Read the model definition and answer for the solid it produces. Units are mm, in the model's axes. Face numbers are marked on the shaded views. A direction names the side the tool comes from. Coordinates: 2 decimals unless noted, no trailing zeros. Loops run counter-clockwise (first coordinate to the right, second up) from the corner with the lowest first, then second, coordinate; pieces in that order, holes last. Notation, with made-up numbers: (-39.75, 20) - (-5.75, 20) arc R17 cw to (-5.75, 51) - close; hole circle Ø11 at (12.25, 83.5). An arc over 180 degrees is marked (long way). Use one line per item in the form item = value. Start each with the question number.
1) The mould has two halves that part along Y. Classify the marked faces 1, 2 and 3: released by +Y, released by -Y, zero draft, split by the parting line, or undercut.
2) A cutting plane is placed at A-A (z = 23). Give the vertices of the cut face in (x, y).
3) Which of the six approach directions +Z, -Z, +X, -X, +Y, -Y give full straight-line access (tool end or side, diameter ignored) to the marked faces 4 and 5?
4) Consider line 1 (Y direction, x = 113, z = 35.5); line 2 (X direction, y = 47.5, z = 35); line 3 (X direction, y = 4.75, z = -17). Determine where each line is inside the solid, lowest interval first.
5) Each of these flat-tipped pins is pushed along its axis until it touches: P1, Ø11, axis at x = 65, y = 74, coming from the +Z side; P2, Ø9.5, axis at x = 125, z = 23, coming from the +Y side; P3, Ø8, axis at x = 17, y = 23.5, coming from the -Z side. Where does it stop, or does it pass through?
6) A cutting plane is placed at D-D (x = 85). Give the vertices of the cut face in (y, z).
7) A cutting plane is placed at C-C (y = 47.5). Give the vertices of the cut face in (x, z), and give its area (3 significant figures).
8) A cutting plane is placed at B-B (x = 113). Give the vertices of the cut face in (y, z), and give its area (3 significant figures).
from build123d import *

# Parameters (mm, degrees)
SKETCH1_R           = 3
SKETCH1_W           = 130
SKETCH1_H           = 10
BOSS_EXTRUDE1_DEPTH = 10
SKETCH2_W           = 130
SKETCH2_H           = 8.023003322
BOSS_EXTRUDE2_DEPTH = 75
SKETCH3_R           = 7.5
SKETCH3_R_2         = 3.5
SKETCH3_R_3         = 10
CUT_EXTRUDE1_DEPTH  = 75
SKETCH4_R           = 3.5
BOSS_EXTRUDE3_DEPTH = 10
SKETCH5_R           = 3.5
CUT_EXTRUDE2_DEPTH  = 10
SKETCH7_W           = 130
SKETCH7_H           = 8.023003322
CUT_EXTRUDE3_DEPTH  = 4
FILLET2_R           = 5
SKETCH8_W           = 4.676136813
SKETCH8_H           = 81
CUT_EXTRUDE4_DEPTH  = 500
SKETCH9_R           = 3
CUT_EXTRUDE5_DEPTH  = 500
SKETCH11_W          = 130
SKETCH11_H          = 10
CUT_EXTRUDE6_DEPTH  = 40
FILLET3_R           = 5
FILLET4_R           = 5
SKETCH12_R          = 3.5
SKETCH12_R_2        = 10
SKETCH12_R_3        = 7.5
BOSS_EXTRUDE4_DEPTH = 1.98


with BuildPart() as part:
    # Sketch1 → Boss-Extrude1 (new body)
    # profile 1 of 3: a face of its own
    with BuildSketch(Plane(origin=(0, 0, 0), x_dir=(1, 0, 0), z_dir=(0, 1, 0))):
        Polygon((0, 63), (0, 0), (5, 0), (130, 0), (130, 63), align=None)
        with Locations(Location((5, 17, 0), (0, 0, 270))):
            Circle(SKETCH1_R, mode=Mode.SUBTRACT)
        with Locations(Location((45, 17, 0), (0, 0, 270))):
            Circle(SKETCH1_R, mode=Mode.SUBTRACT)
        with Locations(Location((5, 57, 0), (0, 0, 270))):
            Circle(SKETCH1_R, mode=Mode.SUBTRACT)
        with Locations(Location((45, 57, 0), (0, 0, 270))):
            Circle(SKETCH1_R, mode=Mode.SUBTRACT)
        with Locations(Location((85, 17, 0), (0, 0, 270))):
            Circle(SKETCH1_R, mode=Mode.SUBTRACT)
        with Locations(Location((125, 17, 0), (0, 0, 270))):
            Circle(SKETCH1_R, mode=Mode.SUBTRACT)
        with Locations(Location((85, 57, 0), (0, 0, 270))):
            Circle(SKETCH1_R, mode=Mode.SUBTRACT)
        with Locations(Location((125, 57, 0), (0, 0, 270))):
            Circle(SKETCH1_R, mode=Mode.SUBTRACT)
    # profile 2 of 3: a face of its own
    with BuildSketch(Plane(origin=(0, 0, 0), x_dir=(1, 0, 0), z_dir=(0, 1, 0))):
        Polygon((5, 0), (0, 0), (0, -27), (130, -27), (130, 0), align=None)
    # profile 3 of 3: a face of its own
    with BuildSketch(Plane(origin=(0, 0, 0), x_dir=(1, 0, 0), z_dir=(0, 1, 0))):
        with Locations((65, -32)):
            Rectangle(SKETCH1_W, SKETCH1_H)
    extrude(amount=BOSS_EXTRUDE1_DEPTH)

    # Sketch2 → Boss-Extrude2 (add)
    with BuildSketch(Plane(origin=(0, 10, 0), x_dir=(1, 0, 0), z_dir=(0, 1, 0))):
        with Locations((65, -32.988498339)):
            Rectangle(SKETCH2_W, SKETCH2_H)
    extrude(amount=BOSS_EXTRUDE2_DEPTH)

    # Sketch3 → Cut-Extrude1 (cut)
    with BuildSketch(Plane(origin=(0, 0, 28.976996678), x_dir=(-1, 0, 0), z_dir=(0, 0, -1))):
        with Locations((-65, 47.5)):
            Circle(SKETCH3_R)
        with Locations((-65, 74)):
            Circle(SKETCH3_R_2)
        with Locations((-17, 71.4)):
            Circle(SKETCH3_R_2)
        with Locations((-17, 23.6)):
            Circle(SKETCH3_R_2)
        with Locations((-17, 47.5)):
            Circle(SKETCH3_R_3)
        with Locations((-65, 21)):
            Circle(SKETCH3_R_2)
        with Locations((-113, 23.6)):
            Circle(SKETCH3_R_2)
        with Locations((-113, 71.4)):
            Circle(SKETCH3_R_2)
        with Locations((-113, 47.5)):
            Circle(SKETCH3_R_3)
    extrude(amount=-CUT_EXTRUDE1_DEPTH, mode=Mode.SUBTRACT)

    # Sketch4 → Boss-Extrude3 (add)
    with BuildSketch(Plane(origin=(0, 0, 28.976996678), x_dir=(-1, 0, 0), z_dir=(0, 0, -1))):
        with Locations((-17, 71.4)):
            Circle(SKETCH4_R)
        with Locations((-17, 23.6)):
            Circle(SKETCH4_R)
        with Locations((-113, 71.4)):
            Circle(SKETCH4_R)
        with Locations((-113, 23.6)):
            Circle(SKETCH4_R)
        with Locations((-65, 74)):
            Circle(SKETCH4_R)
        with Locations((-65, 21)):
            Circle(SKETCH4_R)
    extrude(amount=-BOSS_EXTRUDE3_DEPTH)

    # Sketch5 → Cut-Extrude2 (cut)
    with BuildSketch(Plane(origin=(0, 0, 28.976996678), x_dir=(-1, 0, 0), z_dir=(0, 0, -1))):
        with Locations((-113, 71.5)):
            Circle(SKETCH5_R)
        with Locations((-113, 23.5)):
            Circle(SKETCH5_R)
        with Locations((-17, 71.5)):
            Circle(SKETCH5_R)
        with Locations((-17, 23.5)):
            Circle(SKETCH5_R)
        with Locations((-65, 74)):
            Circle(SKETCH5_R)
        with Locations((-65, 21)):
            Circle(SKETCH5_R)
    extrude(amount=-CUT_EXTRUDE2_DEPTH, mode=Mode.SUBTRACT)

    # Sketch7 → Cut-Extrude3 (cut)
    with BuildSketch(Plane(origin=(0, 85, 0), x_dir=(1, 0, 0), z_dir=(0, 1, 0))):
        with Locations((65, -32.988498339)):
            Rectangle(SKETCH7_W, SKETCH7_H)
    extrude(amount=-CUT_EXTRUDE3_DEPTH, mode=Mode.SUBTRACT)

    # Fillet2
    fillet2_edges = [part.edges().sort_by_distance(p)[0] for p in [
        (130, 5, -63),
        (0, 5, -63),
        (0, 81, 32.988498339),
        (130, 81, 32.988498339),
    ]]
    fillet(fillet2_edges, radius=FILLET2_R)

    # Sketch8 → Cut-Extrude4 (cut)
    with BuildSketch(Plane.ZY):
        with Locations((39.338068406, 40.5)):
            Rectangle(SKETCH8_W, SKETCH8_H)
    extrude(amount=-CUT_EXTRUDE4_DEPTH, mode=Mode.SUBTRACT)

    # Sketch9 → Cut-Extrude5 (cut)
    with BuildSketch(Plane(origin=(0, 10, 0), x_dir=(1, 0, 0), z_dir=(0, 1, 0))):
        with Locations(Location((5, -23, 0), (0, 0, 270))):
            Circle(SKETCH9_R)
        with Locations(Location((45, -23, 0), (0, 0, 270))):
            Circle(SKETCH9_R)
        with Locations(Location((85, -23, 0), (0, 0, 270))):
            Circle(SKETCH9_R)
        with Locations(Location((125, -23, 0), (0, 0, 270))):
            Circle(SKETCH9_R)
    extrude(amount=-CUT_EXTRUDE5_DEPTH, mode=Mode.SUBTRACT)

    # Sketch11 → Cut-Extrude6 (cut)
    with BuildSketch(Plane(origin=(0, 0, -63), x_dir=(-1, 0, 0), z_dir=(0, 0, -1))):
        with Locations((-65, 5)):
            Rectangle(SKETCH11_W, SKETCH11_H)
    extrude(amount=-CUT_EXTRUDE6_DEPTH, mode=Mode.SUBTRACT)

    # Fillet3
    fillet3_edges = [part.edges().sort_by_distance(p)[0] for p in [
        (0, 5, -23),
    ]]
    fillet(fillet3_edges, radius=FILLET3_R)

    # Fillet4
    fillet4_edges = [part.edges().sort_by_distance(p)[0] for p in [
        (130, 5, -23),
    ]]
    fillet(fillet4_edges, radius=FILLET4_R)

    # Sketch12 → Boss-Extrude4 (add)
    # profile 1 of 3: a face of its own
    with BuildSketch(Plane.XY.offset(37)):
        with BuildLine():
            Line((125, 81), (5, 81))
            ThreePointArc((5, 81), (8.535533906, 79.535533906), (10, 76))
            ThreePointArc((10, 76), (5, 71), (0, 76))
            Line((0, 76), (0, 0))
            Line((0, 0), (130, 0))
            Line((130, 0), (130, 76))
            ThreePointArc((130, 76), (121.464466094, 72.464466094), (125, 81))
        make_face()
        with Locations(Location((17, 23.5, 0), (0, 0, 180))):
            Circle(SKETCH12_R, mode=Mode.SUBTRACT)
        with Locations(Location((65, 21, 0), (0, 0, 180))):
            Circle(SKETCH12_R, mode=Mode.SUBTRACT)
        with Locations(Location((113, 23.5, 0), (0, 0, 180))):
            Circle(SKETCH12_R, mode=Mode.SUBTRACT)
        with Locations(Location((17, 47.5, 0), (0, 0, 180))):
            Circle(SKETCH12_R_2, mode=Mode.SUBTRACT)
        with Locations(Location((17, 71.5, 0), (0, 0, 180))):
            Circle(SKETCH12_R, mode=Mode.SUBTRACT)
        with Locations(Location((65, 47.5, 0), (0, 0, 180))):
            Circle(SKETCH12_R_3, mode=Mode.SUBTRACT)
        with Locations(Location((113, 47.5, 0), (0, 0, 180))):
            Circle(SKETCH12_R_2, mode=Mode.SUBTRACT)
        with Locations(Location((65, 74, 0), (0, 0, 180))):
            Circle(SKETCH12_R, mode=Mode.SUBTRACT)
        with Locations(Location((113, 71.5, 0), (0, 0, 180))):
            Circle(SKETCH12_R, mode=Mode.SUBTRACT)
    # profile 2 of 3: a face of its own
    with BuildSketch(Plane.XY.offset(37)):
        with BuildLine():
            ThreePointArc((10, 76), (8.535533906, 79.535533906), (5, 81))
            ThreePointArc((5, 81), (1.464466094, 79.535533906), (0, 76))
            ThreePointArc((0, 76), (5, 71), (10, 76))
        make_face()
    # profile 3 of 3: a face of its own
    with BuildSketch(Plane.XY.offset(37)):
        with BuildLine():
            ThreePointArc((130, 76), (128.535533906, 79.535533906), (125, 81))
            ThreePointArc((125, 81), (121.464466094, 72.464466094), (130, 76))
        make_face()
    extrude(amount=BOSS_EXTRUDE4_DEPTH)


solid = part.part
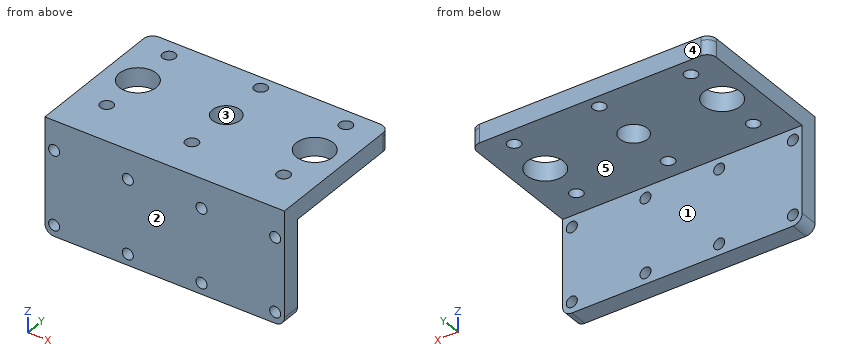
Found:
q1.face_1 = released by +Y
q1.face_2 = released by -Y
q1.face_3 = undercut
q2.outline = (0, 0) - (2, 0) - (2, 10) - (0, 10) - close; (8, 0) - (42, 0) - (42, 10) - (8, 10) - close; (48, 0) - (82, 0) - (82, 10) - (48, 10) - close; (88, 0) - (122, 0) - (122, 10) - (88, 10) - close; (128, 0) - (130, 0) - (130, 10) - (128, 10) - close
q3.face_4 = +Z, -Z, +X, -X, +Y
q3.face_5 = -Z, +X, -X, +Y
q4.line_1 = 0 to 20, 27 to 37.5, 57.5 to 68, 75 to 81
q4.line_2 = 0 to 7, 27 to 57.5, 72.5 to 103, 123 to 130
q4.line_3 = 0 to 2, 8 to 42, 48 to 82, 88 to 122, 128 to 130
q5.P1 = 38.98
q5.P2 = 10
q5.P3 = 28.98
q6.outline = (0, -23) - (10, -23) - (10, -20) - (0, -20) - close; (0, -14) - (10, -14) - (10, 20) - (0, 20) - close; (0, 26) - (10, 26) - (10, 28.98) - (81, 28.98) - (81, 38.98) - (0, 38.98) - close
q7.outline = (0, 28.98) - (7, 28.98) - (7, 38.98) - (0, 38.98) - close; (27, 28.98) - (57.5, 28.98) - (57.5, 38.98) - (27, 38.98) - close; (72.5, 28.98) - (103, 28.98) - (103, 38.98) - (72.5, 38.98) - close; (123, 28.98) - (130, 28.98) - (130, 38.98) - (123, 38.98) - close
q7.area = 750 mm^2
q8.outline = (0, -23) - (10, -23) - (10, 28.98) - (20, 28.98) - (20, 38.98) - (0, 38.98) - close; (27, 28.98) - (37.5, 28.98) - (37.5, 38.98) - (27, 38.98) - close; (57.5, 28.98) - (68, 28.98) - (68, 38.98) - (57.5, 38.98) - close; (75, 28.98) - (81, 28.98) - (81, 38.98) - (75, 38.98) - close
q8.area = 990 mm^2
